Answer from the drawing. Dimensions are ordinates in mm from the lowest x, y and z of the part. Coordinates: 2 decimals unless noted, no trailing zeros. Write each loop counter-clockwise with the first axis right and the second up, starting at its lowest first coordinate (ties: lowest second). Pieces come first, ordered by that corner, then holes.
(1) The part is cut by section B-B on y = 42.5. Determine the outline of the cut face in (x, z) (1 decimal), plus the area to 3 significant figures.
(2) The part is cut by section C-C on z = 62.5. Determine the outline of the cut face in (x, y) (3 decimals), plus the area to 3 significant figures.
(3) Given P1, Ø2, axis at x = 18, z = 37.5, coming from the +Y side; P2, Ø5, axis at x = 3.75, y = 55, coming from the -Z side; P3, Ø2, axis at x = 22.5, z = 15, coming from the +Y side; P4, Ø3, axis at x = 106.25, y = 55, coming from the +Z side, each flat-ended and moving along its own axis, determine where each tip first touches the part or whether it passes through.
(4) Straight lines are drawn through the part: line 1 (Y direction, x = 56.5, z = 17); line 2 (Y direction, x = 81.5, z = 95.5) (1 decimal); line 3 (Z direction, x = 93.5, y = 27). For each, find the intervals that lie inside material, in ascending order.
(5) The part is cut by section A-A on x = 78.5. Determine the outline of the cut face in (y, z).
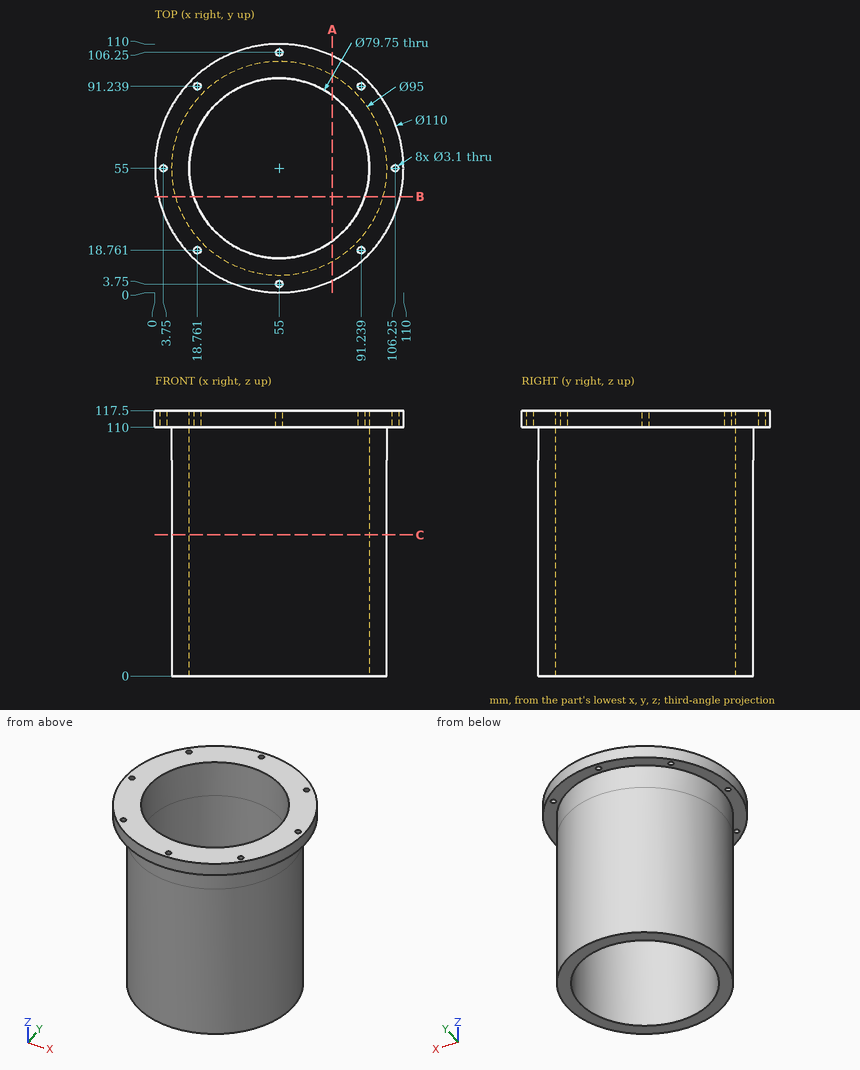
Model answer:
1. outline: (1.4, 110) - (9.2, 110) - (9.2, 0) - (17.1, 0) - (17.1, 117.5) - (1.4, 117.5) - close; (92.9, 0) - (100.8, 0) - (100.8, 110) - (108.6, 110) - (108.6, 117.5) - (92.9, 117.5) - close
1. area: 1,990 mm2
2. outline: circle Ø95 at (55, 55); hole circle Ø79.75 at (55, 55)
2. area: 2,090 mm2
3. P1: stops at y = 85.99
3. P2: stops at z = 110
3. P3: stops at y = 90.55
3. P4: passes through
4. line 1: y = 7.52 to 15.15, 94.85 to 102.48
4. line 2: y = 15.6 to 25.2, 84.8 to 94.4
4. line 3: z = 110 to 117.5
5. outline: (5.27, 110) - (13.72, 110) - (13.72, 0) - (22.79, 0) - (22.79, 117.5) - (5.27, 117.5) - close; (87.21, 0) - (96.28, 0) - (96.28, 110) - (104.73, 110) - (104.73, 117.5) - (87.21, 117.5) - close
